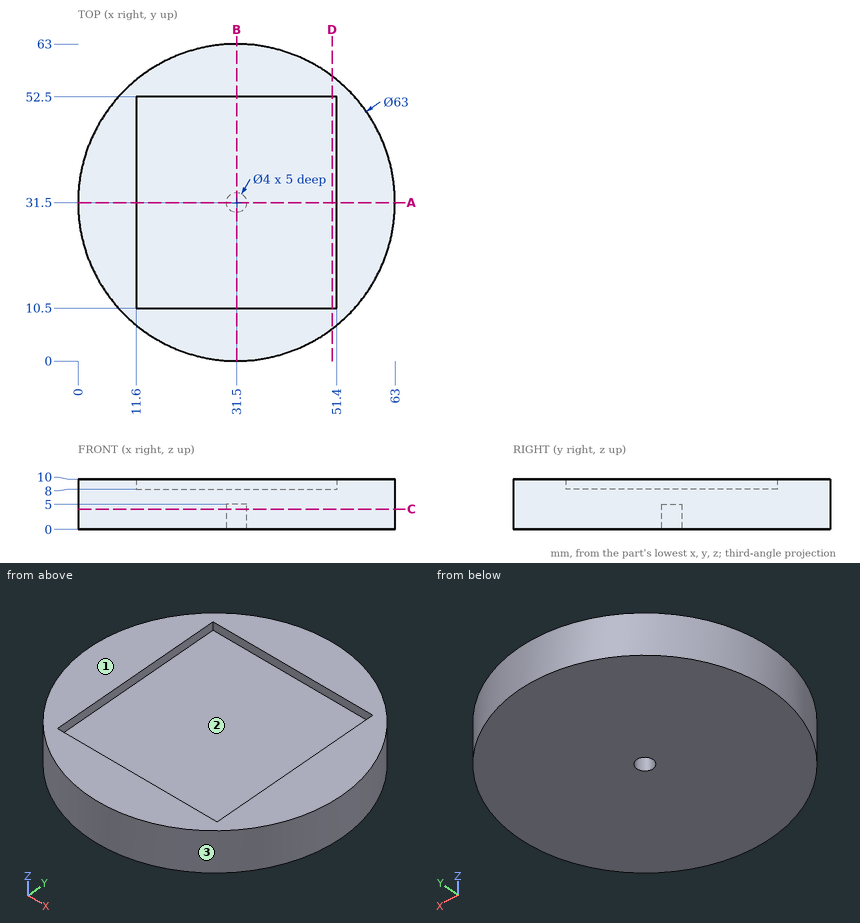
Could you check a few things on this drawing? It's one solid part, dimensions in mm from its lowest x, y, z. Coordinates: 2 decimals unless noted, no trailing zeros. Write each loop counter-clockwise with the first axis right and the second up, starting at its lowest first coordinate (ties: lowest second). Pieces come first, ordered by that corner, then holes.
1) If we section it at A-A (y = 31.5): List the corners of the cut face in (x, z) for me, plus the area to 3 significant figures.
Filled in:
outline: (0, 0) - (29.5, 0) - (29.5, 5) - (33.5, 5) - (33.5, 0) - (63, 0) - (63, 10) - (51.4, 10) - (51.4, 8) - (11.6, 8) - (11.6, 10) - (0, 10) - close
area: 530 mm2
2) Thinking about a two-plate mould opening in X: for the marked faces 1, 2 and 3, which applies, +X half, -X half, draft (parallel to the pull), parting line (faces both ways), or undercut?
Filled in:
face 1: draft
face 2: undercut
face 3: parting line
3) If we section it at C-C (z = 4): List the corners of the cut face in (x, y) for me, plus the area to 3 significant figures.
Filled in:
outline: circle Ø63 at (31.5, 31.5); hole circle Ø4 at (31.5, 31.5)
area: 3,100 mm2
4) I'm going to push flat-ended pins straight in: pin 1 (1.2 mm diameter, centred on x = 31, y = 32, fed in from -Z); pin 2 (3 mm diameter, centred on x = 37, y = 30, fed in from +Z); pin 3 (6 mm diameter, centred on y = 42, z = 3, fed in from -X). Where does each tip first touch, or does it pass through?
Filled in:
pin 1: stops at z = 5
pin 2: stops at z = 8
pin 3: stops at x = 0.91
5) If we section it at B-B (x = 31.5): List the corners of the cut face in (y, z) for me.
Filled in:
outline: (0, 0) - (29.5, 0) - (29.5, 5) - (33.5, 5) - (33.5, 0) - (63, 0) - (63, 10) - (52.5, 10) - (52.5, 8) - (10.5, 8) - (10.5, 10) - (0, 10) - close
6) If I drill on line 1 (Y direction, x = 31.5, z = 1.2); line 2 (Z direction, x = 41, y = 42.5); line 3 (Y direction, x = 41, z = 8.5), over which ranges is the centre line in solid material (lowest first)?
Filled in:
line 1: y = 0 to 29.5, 33.5 to 63
line 2: z = 0 to 8
line 3: y = 1.47 to 10.5, 52.5 to 61.53
7) If we section it at D-D (x = 50.5): List the corners of the cut face in (y, z) for me.
Filled in:
outline: (6.38, 0) - (56.62, 0) - (56.62, 10) - (52.5, 10) - (52.5, 8) - (10.5, 8) - (10.5, 10) - (6.38, 10) - close
